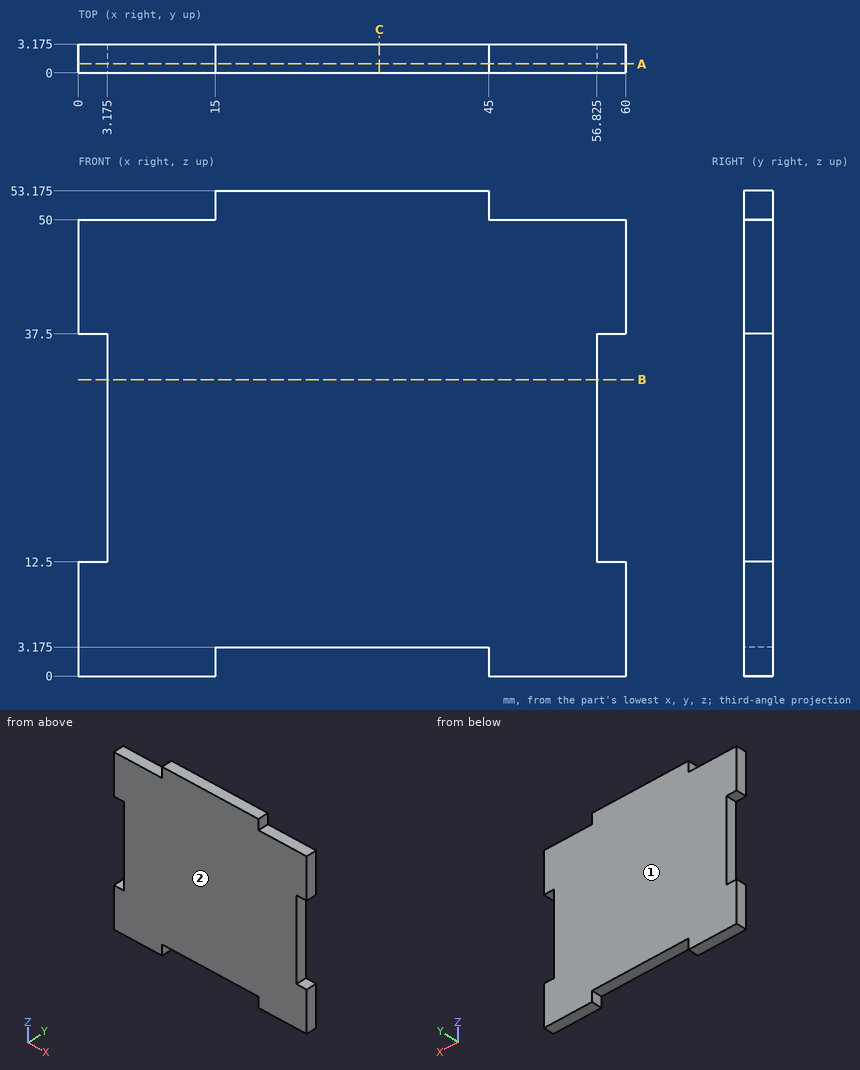
Part print with two shaded views. Sizes in mm from the minimum x, y, z corner. Round coordinates to 2 decimals unless told otherwise and drop trailing zeros. Write each loop counter-clockwise with the first axis right and the second up, starting at its lowest first coordinate (ties: lowest second). Pieces come first, ordered by that corner, then holes. Notation, with made-up numbers: M -24,15 L -8,15 A16 ccw -8,42 Z; hole C 35,-38.75 d5. An arc over 180 degrees is marked long. Answer as CSV lines item,"result". Start each with the question number.
1) Mould opens along Y. For the marked faces 1 and 2 say: +Y half, -Y half, draft (parallel to the pull), parting line (faces both ways), or undercut.
2) Band-saw the part on C-C (x = 33). List the corners of the cut face in (y, z) (3 decimals).
3) Drop flat-ended pins along their axis: pin 1 (1.6 mm diameter, centred on y = 2, z = 52, fed in from +X); pin 2 (1 mm diameter, centred on x = 59, y = 2, fed in from +Z); pin 3 (1 mm diameter, centred on y = 2, z = 26, fed in from +X) (3 decimals). Give the stop position or say it passes through.
4) Band-saw the part on B-B (z = 32.5). List the corners of the cut face in (x, y) (3 decimals).
5) Band-saw the part on A-A (y = 1). List the corners of the cut face in (x, z) (3 decimals).
6) Drill centre lines: L1, parallel to Z at x = 32, y = 0.8 (3 decimals); L2, parallel to Z at x = 48.5, y = 2.4; L3, parallel to X at y = 2.65, z = 35 (3 decimals). Where is each one in solid material? Low to high.
Worked out:
1,face 1,"+Y half"
1,face 2,"-Y half"
2,outline,"M 0,3.175 L 3.175,3.175 L 3.175,53.175 L 0,53.175 Z"
3,pin 1,"x = 45"
3,pin 2,"z = 50"
3,pin 3,"x = 56.825"
4,outline,"M 3.175,0 L 56.825,0 L 56.825,3.175 L 3.175,3.175 Z"
5,outline,"M 0,0 L 15,0 L 15,3.175 L 45,3.175 L 45,0 L 60,0 L 60,12.5 L 56.825,12.5 L 56.825,37.5 L 60,37.5 L 60,50 L 45,50 L 45,53.175 L 15,53.175 L 15,50 L 0,50 L 0,37.5 L 3.175,37.5 L 3.175,12.5 L 0,12.5 Z"
6,L1,"3.175 to 53.175"
6,L2,"0 to 50"
6,L3,"3.175 to 56.825"
